Can you work these out from the model? Positions are in its coordinate system, mm. Face numbers are marked on the shaded views. A direction names the side the tool comes from. Give positions to 0.01 mm unless a question says otherwise; leave off trailing zeros. Loops run counter-clockwise (first coordinate to the right, second up) from the corner with the lowest first, then second, coordinate; pieces in that order, holes last. Notation, with made-up numbers: (74, 31) - (88, 31) arc R14 ccw to (88, 39) - close; hole circle Ø8 at (88.5, 5). An arc over 180 degrees is marked (long way). Answer as a JSON object with one key per item and string values.
```python
from build123d import *

# Parameters (mm, degrees)
F0_W     = 80
F0_H     = 50
F1_DEPTH = 33.8
F2_R     = 25
F3_DEPTH = 104.1
F4_R     = 10
F5_W     = 60
F5_H     = 42.5
F5_H_2   = 7.5
F6_DEPTH = 26.5
F7_SIZE  = 10


with BuildPart() as f1:
    # F0 (on Front) → F1 (new body, symmetric)
    with BuildSketch(Plane.XZ):
        Rectangle(F0_W, F0_H)
    extrude(amount=F1_DEPTH, both=True)

    # F2 (on face) → F3 (cut)
    with BuildSketch(Plane.XY.offset(25)):
        Circle(F2_R)
    extrude(amount=-F3_DEPTH, mode=Mode.SUBTRACT)

    # F4
    f4_edges = [f1.edges().sort_by_distance(p)[0] for p in [
        (40, -33.8, 0),
        (-40, -33.8, 0),
    ]]
    fillet(f4_edges, radius=F4_R)

    # F5 (on face) → F6 (cut)
    with BuildSketch(Plane(origin=(0, 33.8, 0), x_dir=(-1, 0, 0), z_dir=(0, 1, 0))):
        with Locations((0, -3.75)):
            Rectangle(F5_W, F5_H)
        with Locations((0, -28.75)):
            Rectangle(F5_W, F5_H_2)
    extrude(amount=-F6_DEPTH, mode=Mode.SUBTRACT)

    # F7
    f7_edges = [f1.edges().sort_by_distance(p)[0] for p in [
        (26.955229, 7.3, 17.5),
        (-26.955229, 7.3, 17.5),
    ]]
    chamfer(f7_edges, length=F7_SIZE)


solid = f1.part
```
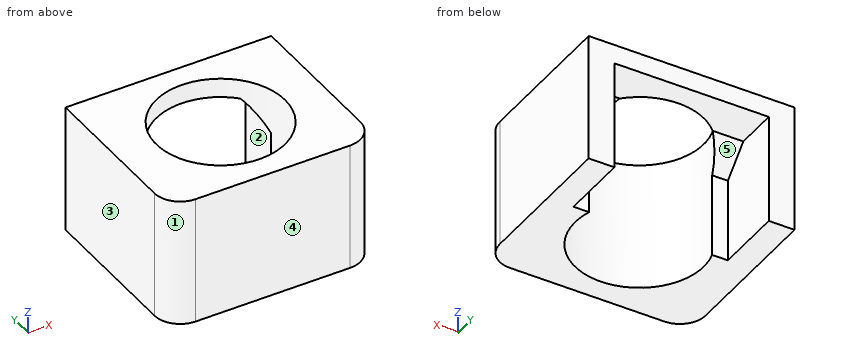
1) Which directions (+Z, -Z, +X, -X, +Y, -Y) give clear straight access to the entire face, cutting with the end or side of a thin tool? Please do the marked faces 1 and 2.
Check sheet entries:
{"face 1": "+Z, -Z, -X, -Y", "face 2": "-Z, +Y"}
2) Imagine slicing it at C-C on x = -26. Write out the boundary of the cut face in (y, z), and give its area (3 significant figures).
Check sheet entries:
{"outline": "(-33.8, -25) - (7.3, -25) - (7.3, 7.5) - (17.3, 17.5) - (33.8, 17.5) - (33.8, 25) - (-33.8, 25) - close", "area": "2,300 mm2"}
3) If we mould it in two halves opening along X, with no side actions, what happens to the marked faces 3, 4 and 5? For each: released by +X, released by -X, zero draft, split by the parting line, or undercut.
Check sheet entries:
{"face 3": "released by -X", "face 4": "zero draft", "face 5": "undercut"}
4) I'm going to push flat-ended pins straight in: P1, Ø2, axis at x = 18.5, z = -13.5, coming from the +Y side; P2, Ø4, axis at x = 3, z = -14, coming from the +Y side; P3, Ø5, axis at x = -12.5, y = 23, coming from the -Z side. Where does each tip first touch, or does it pass through?
Check sheet entries:
{"P1": "y = -15.64", "P2": "y = -24.49", "P3": "z = 17.5"}
5) Imagine slicing it at B-B on y = 0. Write out the boundary of the cut face in (x, z).
Check sheet entries:
{"outline": "(-40, -25) - (-25, -25) - (-25, 25) - (-40, 25) - close; (25, -25) - (40, -25) - (40, 25) - (25, 25) - close"}
6) Imagine slicing it at A-A on x = 0. Write out the boundary of the cut face in (y, z), and give its area (3 significant figures).
Check sheet entries:
{"outline": "(-33.8, -25) - (-25, -25) - (-25, 25) - (-33.8, 25) - close; (25, 17.5) - (33.8, 17.5) - (33.8, 25) - (25, 25) - close", "area": "506 mm2"}
7) I need wall thicknesses on L1, parallel to X at y = 0, z = 6.5; L2, parallel to X at y = 18, z = 14; L3, parallel to Y at x = 0, z = -8. Which ranges of each line are inside material? Lowest first, please.
Check sheet entries:
{"L1": "-40 to -25, 25 to 40", "L2": "-40 to -30, 30 to 40", "L3": "-33.8 to -25"}
8) Imagine slicing it at D-D on z = -6. Write out the boundary of the cut face in (x, y), and give its area (3 significant figures).
Check sheet entries:
{"outline": "(-40, -23.8) arc R10 ccw to (-30, -33.8) - (30, -33.8) arc R10 ccw to (40, -23.8) - (40, 33.8) - (30, 33.8) - (30, 7.3) - (23.91, 7.3) arc R25 cw (long way) to (-23.91, 7.3) - (-30, 7.3) - (-30, 33.8) - (-40, 33.8) - close", "area": "2,430 mm2"}
